```python
from build123d import *

# Parameters (mm, degrees)
BOSS_EXTRUDE2_DEPTH = 38.1
SKETCH1_W           = 25.35
SKETCH1_H           = 29.67
BOSS_EXTRUDE3_DEPTH = 3.81
SKETCH3_W           = 3
SKETCH3_H           = 7.62
CUT_EXTRUDE1_DEPTH  = 4.81
SKETCH4_W           = 7.62
SKETCH4_H           = 30.1
CUT_EXTRUDE2_DEPTH  = 4.81
SKETCH5_R           = 1.5
CUT_EXTRUDE3_DEPTH  = 4.81
SKETCH6_R           = 1.45
CUT_EXTRUDE4_DEPTH  = 24.844
FILLET1_R           = 4
FILLET4_R           = 2.54
FILLET2_R           = 1.016
FILLET3_R           = 1.27
FILLET5_R           = 1.016
CUT_EXTRUDE5_DEPTH  = 1.27


with BuildPart() as part:
    # Sketch2 → Boss-Extrude2 (new body)
    with BuildSketch(Plane(origin=(0, 0, 0), x_dir=(1, 0, 0), z_dir=(0, 1, 0))):
        Polygon((-9.5, -11.43), (9.5, -11.43), (9.5, -5.08), (12.04, -5.08), (12.04, -14.43), (-13.31, -14.43), (-13.31, 15.24), (12.04, 15.24), (12.04, 7.62), (9.5, 7.62), (9.5, 11.43), (-9.5, 11.43), align=None)
    extrude(amount=BOSS_EXTRUDE2_DEPTH)

    # Sketch1 → Boss-Extrude3 (add)
    with BuildSketch(Plane(origin=(0, 0, 0), x_dir=(1, 0, 0), z_dir=(0, 1, 0))):
        with Locations((-0.635, 0.405)):
            Rectangle(SKETCH1_W, SKETCH1_H)
    extrude(amount=-BOSS_EXTRUDE3_DEPTH)

    # Sketch3 → Cut-Extrude1 (cut, through all)
    with BuildSketch(Plane(origin=(0, 0, 0), x_dir=(1, 0, 0), z_dir=(0, 1, 0))):
        with Locations((-0.38, 0)):
            Rectangle(SKETCH3_W, SKETCH3_H)
    extrude(amount=-CUT_EXTRUDE1_DEPTH, mode=Mode.SUBTRACT)

    # Sketch4 → Cut-Extrude2 (cut, through all)
    with BuildSketch(Plane(origin=(-9.5, 0, 0), x_dir=(0, 0, -1), z_dir=(1, 0, 0))):
        with Locations((0, 23.05)):
            Rectangle(SKETCH4_W, SKETCH4_H)
    extrude(amount=-CUT_EXTRUDE2_DEPTH, mode=Mode.SUBTRACT)

    # Sketch5 → Cut-Extrude3 (cut, through all)
    with BuildSketch(Plane(origin=(-9.5, 0, 0), x_dir=(0, 0, -1), z_dir=(1, 0, 0))):
        with Locations((-9.1700096, 31)):
            Circle(SKETCH5_R)
        with Locations((8.2299904, 31)):
            Circle(SKETCH5_R)
    extrude(amount=-CUT_EXTRUDE3_DEPTH, mode=Mode.SUBTRACT)

    # Sketch6 → Cut-Extrude4 (cut)
    with BuildSketch(Plane.XY.offset(14.43)):
        with Locations((-11.405, 19.05)):
            Circle(SKETCH6_R)
        with Locations((-3.81, -1.905)):
            Circle(SKETCH6_R)
    extrude(amount=-CUT_EXTRUDE4_DEPTH, mode=Mode.SUBTRACT)

    # Fillet1
    fillet1_edges = [part.edges().sort_by_distance(p)[0] for p in [
        (0, 0, -11.43),
        (0, 0, 11.43),
    ]]
    fillet(fillet1_edges, radius=FILLET1_R)


with BuildPart() as body_2:
    # Mirror1: mirrored copy
    add(part.part.mirror(Plane.XY))

    # Fillet4
    fillet4_edges = [body_2.edges().sort_by_distance(p)[0] for p in [
        (-11.405, 8, -3.81),
        (-11.405, 8, 3.81),
    ]]
    fillet(fillet4_edges, radius=FILLET4_R)

    # Fillet2
    fillet2_edges = [body_2.edges().sort_by_distance(p)[0] for p in [
        (-13.31, 17.145, 15.24),
        (12.04, 17.145, 15.24),
        (12.04, -3.81, 0.405),
        (-13.31, -3.81, 0.405),
        (-0.635, -3.81, 15.24),
        (12.04, 38.1, 11.43),
        (-0.635, 38.1, 15.24),
        (-13.31, 38.1, 9.525),
        (-13.31, 38.1, -9.12),
        (-11.405, 38.1, -3.81),
        (-11.405, 38.1, 3.81),
    ]]
    fillet(fillet2_edges, radius=FILLET2_R)

    # Fillet3
    fillet3_edges = [body_2.edges().sort_by_distance(p)[0] for p in [
        (-1.88, 0, 0),
        (-0.38, 0, -3.81),
        (1.12, 0, 0),
        (-0.38, 0, 3.81),
    ]]
    fillet(fillet3_edges, radius=FILLET3_R)

    # Fillet5
    fillet5_edges = [body_2.edges().sort_by_distance(p)[0] for p in [
        (12.04, 38.1, -9.755),
        (10.77, 38.1, -5.08),
    ]]
    fillet(fillet5_edges, radius=FILLET5_R)

    # Sketch7 → Cut-Extrude5 (cut)
    with BuildSketch(Plane(origin=(0, 0, 0), x_dir=(1, 0, 0), z_dir=(0, 1, 0))):
        Polygon((4.129986879, -2.992887734), (4.129986879, -2.328037307), (10.778491153, -2.328037307), (10.778491153, 0.521321667), (11.538320213, 0.521321667), (11.538320213, -2.992887734), align=None)
        Polygon((3.940029614, 2.230937052), (3.940029614, 2.895787479), (6.124538161, 2.895787479), (6.124538161, 3.845573804), (6.789388589, 3.845573804), (6.789388589, 2.895787479), (11.538320213, 2.895787479), (11.538320213, 2.230937052), (6.789388589, 2.230937052), (6.789388589, 1.281150727), (6.124538161, 1.281150727), (6.124538161, 2.230937052), align=None)
    extrude(amount=-CUT_EXTRUDE5_DEPTH, mode=Mode.SUBTRACT)


solid = body_2.part
```
Here's how the part is built. I have some questions about the finished solid (model axes, mm). A direction names the side the tool comes from. Round coordinates to 2 decimals unless told otherwise and drop trailing zeros. Write each loop counter-clockwise with the first axis right and the second up, starting at its lowest first coordinate (ties: lowest second). Pieces come first, ordered by that corner, then holes.
Q1. If we section it at D-D on x = -10.5: Write out the boundary of the cut face in (y, z).
Q2. Please list where these lines run through material, in increasing order: probe 1 along X at (y, z) = (17, -6.5); probe 2 along Z at (x, y) = (7.5, 19.5); probe 3 along Z at (x, y) = (10.25, 23.5).
Q3. If we mould it in two halves opening along Y, with no side actions, what happens to faces 1 (the flat face through (-4, -2, 10.414)), 2 (the cylindrical face through (-10.625, 20.273, -9.194)), 3 (the cylindrical face through (-11.432, 8.764, 3.086)), 4 (the flat face through (-1, 17, 15.24))? For each: +Y half, -Y half, draft (parallel to the pull), parting line (faces both ways), or undercut.
Q4. If we section it at A-A on z = 0: Give the number of separate pieces and of enclosed holes in the cut face, plus the area to 3 significant figures.
Q5. Which directions (+Z, -Z, +X, -X, +Y, -Y) give clear straight access to the entire face, cutting with the end or side of a thin tool? Please do faces 5 (the flat face through (-11, 24, -3.81)), 6 (the flat face through (9, -1, -2.231)), 7 (the flat face through (-1, 17, -14.43)), 8 (the flat face through (1.12, -3, 0)), 9 (the flat face through (-11, 19, 10.414)).
Q6. If we section it at C-C on y = 25: Write out the boundary of the cut face in (x, z), plus the area to 3 significant figures.
Q7. Will these pins go through, and if not, where does the flat tip stop? P1, Ø4, axis at y = 22, z = 2.5, coming from the +X side; P2, Ø0.8, axis at x = -11.5, z = -0.5, coming from the +Y side.
Q8. If we section it at B-B on y = 31: Write out the boundary of the cut face in (x, z), plus the area to 3 significant figures.
Answer below:
1. outline: (-3.81, -14.43) - (17.92, -14.43) - (17.92, -3.81) - (10.54, -3.81) arc R2.54 cw to (8, -1.27) - (8, 1.27) arc R2.54 cw to (10.54, 3.81) - (17.92, 3.81) - (17.92, 10.41) - (20.18, 10.41) - (20.18, 3.81) - (37.08, 3.81) arc R1.02 ccw to (38.1, 4.83) - (38.1, 14.22) arc R1.02 ccw to (37.08, 15.24) - (-2.79, 15.24) arc R1.02 ccw to (-3.81, 14.22) - close; (20.18, -14.43) - (38.1, -14.43) - (38.1, -4.83) arc R1.02 ccw to (37.08, -3.81) - (20.18, -3.81) - close; hole circle Ø3 at (31, -9.17); hole circle Ø3 at (31, 8.23)
2. probe 1: x = -13.31 to -9.5, 9.5 to 12.04
2. probe 2: z = -14.43 to -11.43, 11.43 to 15.24
2. probe 3: z = -14.43 to -5.08, 7.62 to 15.24
3. face 1: undercut
3. face 2: undercut
3. face 3: +Y half
3. face 4: draft
4. separate pieces: 2
4. enclosed holes: 1
4. area: 107 mm2
5. face 5: +X, -X, +Y
5. face 6: +Y
5. face 7: -Z, +X, -X, +Y, -Y
5. face 8: +Y, -Y
5. face 9: -Z
6. outline: (-13.31, -14.43) - (12.04, -14.43) - (12.04, -5.08) - (9.5, -5.08) - (9.5, -11.43) - (-9.5, -11.43) - (-9.5, -3.81) - (-13.31, -3.81) - close; (-13.31, 3.81) - (-9.5, 3.81) - (-9.5, 11.43) - (9.5, 11.43) - (9.5, 7.62) - (12.04, 7.62) - (12.04, 14.22) arc R1.02 ccw to (11.02, 15.24) - (-12.29, 15.24) arc R1.02 ccw to (-13.31, 14.22) - close
6. area: 256 mm2
7. P1: stops at x = -9.5
7. P2: stops at y = 8
8. outline: (-13.31, -14.43) - (12.04, -14.43) - (12.04, -5.08) - (9.5, -5.08) - (9.5, -11.43) - (-9.5, -11.43) - (-9.5, -10.67) - (-13.31, -10.67) - close; (-13.31, -7.67) - (-9.5, -7.67) - (-9.5, -3.81) - (-13.31, -3.81) - close; (-13.31, 3.81) - (-9.5, 3.81) - (-9.5, 6.73) - (-13.31, 6.73) - close; (-13.31, 9.73) - (-9.5, 9.73) - (-9.5, 11.43) - (9.5, 11.43) - (9.5, 7.62) - (12.04, 7.62) - (12.04, 14.22) arc R1.02 ccw to (11.02, 15.24) - (-12.29, 15.24) arc R1.02 ccw to (-13.31, 14.22) - close
8. area: 233 mm2
